Check sheet for the modelled part. Datum: model origin and axes. Units: mm. A direction names the side the tool comes from. Give positions to 0.01 mm unless a question says otherwise; leave off trailing zeros. Order: outer loops, then holes, each group sorted by start corner. A loop starts at its lowest first (then second) coordinate and runs counter-clockwise, first axis right, second up.
Item 1: Release check for a two-part mould opening along X. For faces 1 (the flat face through (34, 21, -12)), 2 (the cylindrical face through (15.02, 23.03, 47.69)), 3 (the cylindrical face through (25.48, -2.02, 0.33)) record: released by +X, released by -X, zero draft, split by the parting line, or undercut.
Item 2: Gauge pin test, flat ends, axial feed: P1, Ø1, axis at x = -30, y = 16, coming from the -Z side; P2, Ø1, axis at x = -24, z = -9, coming from the +Y side; P3, Ø1.5, axis at y = 5, z = -1, coming from the +X side. Record the tip position at first contact, or that the pin passes through.
Item 3: Sectioned sample at C-C on y = 22.75. Record the boundary of the cut face in (x, z), and give its area (3 significant figures).
Item 4: Access from +Z, -Z, +X, -X, +Y, -Y to the whole of each face (thin tool, end or side, straight path). Record for faces 4 (the cylindrical face through (-1.32, 12.68, 29.97)), 5 (the cylindrical face through (-12.621, -2.015, -16.126)), 6 (the cylindrical face through (-21, 9, -28)).
Item 5: Sectioned sample at D-D on x = 0. Count the separate pieces of the cut face and the enclosed holes in it, and give its area (3 significant figures).
Item 6: Sectioned sample at B-B on x = 40. Record the boundary of the cut face in (y, z) (3 decimals), and give its area (3 significant figures).
Item 7: Material ranges on line 1 along X through (y, z) = (-3.05, 0); line 2 along X through (y, z) = (23.35, 0); line 3 along Y through (x, z) = (-37.5, 26), recorded low to high.
Item 8: Sectioned sample at A-A on z = 40. Record the boundary of the cut face in (x, y) (3 decimals), and give its area (3 significant figures).
from build123d import *

# Parameters (mm, degrees)
SKETCH1_R                        = 35
SKETCH1_R_2                      = 13
BOSS_EXTRUDE1_DEPTH              = 4
F_5_0_MM_DOWEL_HOLES1_AT_2_COUNT = 2
F_5_0_MM_DOWEL_HOLES1_AT_2_PITCH = 32.526911935
F_5_0_MM_DOWEL_HOLES2_AT_2_COUNT = 2
F_5_0_MM_DOWEL_HOLES2_AT_2_PITCH = 28.284271247
BOSS_EXTRUDE2_START              = 21
SKETCH6_R                        = 35
SKETCH6_R_2                      = 30
BOSS_EXTRUDE2_DEPTH              = 21
BOSS_EXTRUDE3_START              = 4
SKETCH7_R                        = 50
SKETCH7_R_2                      = 30
BOSS_EXTRUDE3_DEPTH              = 4
F_8_0_MM_DOWEL_HOLES1_AT_2_COUNT = 2
F_8_0_MM_DOWEL_HOLES1_AT_2_PITCH = 56.568542495


with BuildPart() as part:
    # Sketch1 → Boss-Extrude1 (new body)
    with BuildSketch(Plane(origin=(0, 0, 0), x_dir=(1, 0, 0), z_dir=(0, 1, 0))):
        with Locations(Location((0, 0, 0), (0, 0, 270))):
            Circle(SKETCH1_R)
        with Locations(Location((0, 0, 0), (0, 0, 270))):
            Circle(SKETCH1_R_2, mode=Mode.SUBTRACT)
    extrude(amount=-BOSS_EXTRUDE1_DEPTH)

    # Sketch3 → Ø5.0 mm Dowel Holes1 (revolve, cut)
    with BuildSketch(Plane(origin=(0, -4, 23), x_dir=(0, 0, -1), z_dir=(1, 0, 0))):
        Polygon((0, 0), (0, 21.502151548), (2.5, 20), (2.5, 0.025), (2.525, 0), align=None)
    f_5_0_mm_dowel_holes1 = revolve(axis=Axis((0, -10.35, 23), (0, 1, 0)), mode=Mode.SUBTRACT)

    # Ø5.0 mm Dowel Holes1 at 2: Ø5.0 mm Dowel Holes1 ×2
    with Locations(*[Vector(-0.7071067811865476, 0, -0.7071067811865476) * (i * F_5_0_MM_DOWEL_HOLES1_AT_2_PITCH) for i in range(1, F_5_0_MM_DOWEL_HOLES1_AT_2_COUNT)]):
        add(f_5_0_mm_dowel_holes1, mode=Mode.SUBTRACT)

    # Mirror1: Ø5.0 mm Dowel Holes1 across plane
    add(f_5_0_mm_dowel_holes1.mirror(Plane(origin=(0, 0, 0), x_dir=(0, 0, 1), z_dir=(1, 0, 0))), mode=Mode.SUBTRACT)

    # Mirror1 copy 1 sketch → Mirror1 copy 1 (revolve, cut)
    with BuildSketch(Plane(origin=(23, -4, 0), x_dir=(0, 0, -1), z_dir=(-1, 0, 0))):
        Polygon((0, 0), (0, -21.502151548), (2.5, -20), (2.5, -0.025), (2.525, 0), align=None)
    revolve(axis=Axis((23, -10.35, 0), (0, -1, 0)), mode=Mode.SUBTRACT)

    # Mirror1 at the second plane: Ø5.0 mm Dowel Holes1 across plane
    add(f_5_0_mm_dowel_holes1.mirror(Plane.XY), mode=Mode.SUBTRACT)

    # Mirror1 at the second plane copy 1 sketc → Mirror1 at the second plane copy 1 (revolve, cut)
    with BuildSketch(Plane(origin=(-23, -4, 0), x_dir=(0, 0, 1), z_dir=(1, 0, 0))):
        Polygon((0, 0), (0, -21.502151548), (2.5, -20), (2.5, -0.025), (2.525, 0), align=None)
    revolve(axis=Axis((-23, -10.35, 0), (0, -1, 0)), mode=Mode.SUBTRACT)

    # Sketch5 → Ø5.0 mm Dowel Holes2 (revolve, cut)
    with BuildSketch(Plane(origin=(-14.142135624, -4, 14.142135624), x_dir=(0, 0, -1), z_dir=(1, 0, 0))):
        Polygon((0, 0), (0, 21.502151548), (2.5, 20), (2.5, 0.025), (2.525, 0), align=None)
    f_5_0_mm_dowel_holes2 = revolve(axis=Axis((-14.142135624, -10.35, 14.142135624), (0, 1, 0)), mode=Mode.SUBTRACT)

    # Ø5.0 mm Dowel Holes2 at 2: Ø5.0 mm Dowel Holes2 ×2
    with Locations(*[(i * F_5_0_MM_DOWEL_HOLES2_AT_2_PITCH, 0, 0) for i in range(1, F_5_0_MM_DOWEL_HOLES2_AT_2_COUNT)]):
        add(f_5_0_mm_dowel_holes2, mode=Mode.SUBTRACT)

    # Mirror2: Ø5.0 mm Dowel Holes2 across plane
    add(f_5_0_mm_dowel_holes2.mirror(Plane.XY), mode=Mode.SUBTRACT)

    # Mirror2 copy 1 sketch → Mirror2 copy 1 (revolve, cut)
    with BuildSketch(Plane(origin=(14.142135624, -4, -14.142135624), x_dir=(0, 0, 1), z_dir=(1, 0, 0))):
        Polygon((0, 0), (0, -21.502151548), (2.5, -20), (2.5, -0.025), (2.525, 0), align=None)
    revolve(axis=Axis((14.142135624, -10.35, -14.142135624), (0, -1, 0)), mode=Mode.SUBTRACT)

    # Sketch6 → Boss-Extrude2 (add)
    with BuildSketch(Plane(origin=(0, 0, 0), x_dir=(1, 0, 0), z_dir=(0, 1, 0)).offset(BOSS_EXTRUDE2_START)):
        with Locations(Location((0, 0, 0), (0, 0, 270))):
            Circle(SKETCH6_R)
        with Locations(Location((0, 0, 0), (0, 0, 90))):
            Circle(SKETCH6_R_2, mode=Mode.SUBTRACT)
    extrude(amount=-BOSS_EXTRUDE2_DEPTH)

    # Sketch7 → Boss-Extrude3 (add)
    with BuildSketch(Plane(origin=(0, 21, 0), x_dir=(1, 0, 0), z_dir=(0, 1, 0)).offset(BOSS_EXTRUDE3_START)):
        with Locations(Location((0, 0, 0), (0, 0, 270))):
            Circle(SKETCH7_R)
        with Locations(Location((0, 0, 0), (0, 0, 90))):
            Circle(SKETCH7_R_2, mode=Mode.SUBTRACT)
    extrude(amount=-BOSS_EXTRUDE3_DEPTH)

    # Sketch9 → Ø8.0 mm Dowel Holes1 (revolve, cut)
    with BuildSketch(Plane(origin=(0, 25, -40), x_dir=(0, 0, 1), z_dir=(1, 0, 0))):
        Polygon((0, 0), (0, 22.403442476), (4, 20), (4, 0.025), (4.025, 0), align=None)
    f_8_0_mm_dowel_holes1 = revolve(axis=Axis((0, 31.35, -40), (0, -1, 0)), mode=Mode.SUBTRACT)

    # Ø8.0 mm Dowel Holes1 at 2: Ø8.0 mm Dowel Holes1 ×2
    with Locations(*[Vector(-0.7071067811865476, 0, 0.7071067811865476) * (i * F_8_0_MM_DOWEL_HOLES1_AT_2_PITCH) for i in range(1, F_8_0_MM_DOWEL_HOLES1_AT_2_COUNT)]):
        add(f_8_0_mm_dowel_holes1, mode=Mode.SUBTRACT)

    # Mirror3: Ø8.0 mm Dowel Holes1 across plane
    add(f_8_0_mm_dowel_holes1.mirror(Plane(origin=(0, 0, 0), x_dir=(0, 0, 1), z_dir=(1, 0, 0))), mode=Mode.SUBTRACT)

    # Mirror3 copy 1 sketch → Mirror3 copy 1 (revolve, cut)
    with BuildSketch(Plane(origin=(40, 25, 0), x_dir=(0, 0, 1), z_dir=(-1, 0, 0))):
        Polygon((0, 0), (0, -22.403442476), (4, -20), (4, -0.025), (4.025, 0), align=None)
    revolve(axis=Axis((40, 31.35, 0), (0, 1, 0)), mode=Mode.SUBTRACT)

    # Mirror3 at the second plane: Ø8.0 mm Dowel Holes1 across plane
    add(f_8_0_mm_dowel_holes1.mirror(Plane.XY), mode=Mode.SUBTRACT)

    # Mirror3 at the second plane copy 1 sketc → Mirror3 at the second plane copy 1 (revolve, cut)
    with BuildSketch(Plane(origin=(-40, 25, 0), x_dir=(0, 0, -1), z_dir=(1, 0, 0))):
        Polygon((0, 0), (0, -22.403442476), (4, -20), (4, -0.025), (4.025, 0), align=None)
    revolve(axis=Axis((-40, 31.35, 0), (0, 1, 0)), mode=Mode.SUBTRACT)


solid = part.part
Report:
1. face 1: zero draft
1. face 2: split by the parting line
1. face 3: undercut
2. P1: stops at z = -18.83
2. P2: stops at y = 0
2. P3: stops at x = 35
3. outline: circle Ø100 at (0, 0); hole circle Ø8 at (-40, 0); hole circle Ø60 at (0, 0); hole circle Ø8 at (0, -40); hole circle Ø8 at (0, 40); hole circle Ø8 at (40, 0)
3. area: 4,830 mm2
4. face 4: +Y
4. face 5: +Y, -Y
4. face 6: -Y
5. separate pieces: 6
5. enclosed holes: 0
5. area: 442 mm2
6. outline: (21, -30) - (25, -30) - (25, -4.025) - (24.975, -4) - (21, -4) - close; (21, 4) - (24.975, 4) - (25, 4.025) - (25, 30) - (21, 30) - close
6. area: 208 mm2
7. line 1: x = -35 to -25.5, -20.5 to -13, 13 to 20.5, 25.5 to 35
7. line 2: x = -50 to -44, -36 to -30, 30 to 36, 44 to 50
7. line 3: y = 21 to 25
8. outline: (-30, 21) - (-4, 21) - (-4, 24.975) - (-4.025, 25) - (-30, 25) - close; (4, 21) - (30, 21) - (30, 25) - (4.025, 25) - (4, 24.975) - close
8. area: 208 mm2
